```python
from build123d import *

# Parameters (mm, degrees)
SKETCH1_R               = 1.6
BOSS_EXTRUDE1_DEPTH     = 6
SALIENTE_EXTRUIR1_DEPTH = 7


with BuildPart() as part:
    # Sketch1 → Boss-Extrude1 (new body)
    # profile 1 of 2: a face of its own
    with BuildSketch(Plane.XY):
        with BuildLine():
            Line((31.98, 5), (0, 5))
            ThreePointArc((0, 5), (-5, 0), (0, -5))
            Line((0, -5), (33.93, -5))
            Line((33.93, -5), (37.237412205, -3.749803263))
            ThreePointArc((37.237412205, -3.749803263), (38.607019153, 1.767906062), (33.93, 5))
            Line((33.93, 5), (31.98, 5))
        make_face()
        Circle(SKETCH1_R, mode=Mode.SUBTRACT)
        with Locations((33.93, 0)):
            Circle(SKETCH1_R, mode=Mode.SUBTRACT)
    # profile 2 of 2: a face of its own
    with BuildSketch(Plane.XY):
        with BuildLine():
            Line((83.410038042, 35.902284495), (31.98, 5))
            Line((31.98, 5), (33.93, 5))
            ThreePointArc((33.93, 5), (38.607019153, 1.767906062), (37.237412205, -3.749803263))
            Line((37.237412205, -3.749803263), (88.667450247, 27.152481232))
            Line((88.667450247, 27.152481232), (83.410038042, 35.902284495))
        make_face()
    extrude(amount=BOSS_EXTRUDE1_DEPTH)

    # Croquis3 → Saliente-Extruir1 (add)
    with BuildSketch(Plane.XY.offset(6)):
        Polygon((83.410038042, 35.902284495), (88.667450247, 27.152481232), (54.380758219, 6.550958236), (49.123346014, 15.300761498), align=None)
    extrude(amount=SALIENTE_EXTRUIR1_DEPTH)


solid = part.part
```
Check sheet for the modelled part. Datum: model origin and axes. Units: mm. A direction names the side the tool comes from. Give positions to 0.01 mm unless a question says otherwise; leave off trailing zeros. Write each loop counter-clockwise with the first axis right and the second up, starting at its lowest first coordinate (ties: lowest second). Pieces come first, ordered by that corner, then holes.
Item 1: Cross-section at A-A (z = 3). Enter the section's corners in (x, y), and give its area (3 significant figures).
Item 2: Gauge pin test, flat ends, axial feed: pin 1 (3 mm diameter, centred on y = 30, z = 11.5, fed in from -X); pin 2 (2 mm diameter, centred on y = 19.5, z = 9, fed in from +X); pin 3 (16 mm diameter, centred on x = 35.5, y = 0.5, fed in from +Z). Record the tip position at first contact, or that the pin passes through.
Item 3: Cross-section at C-C (z = 9). Enter the section's corners in (x, y), and give its area (3 significant figures).
Item 4: Access from +Z, -Z, +X, -X, +Y, -Y to the whole of each face (thin tool, end or side, straight path). Record for faces 4 (the face through (69, 21, 13)), 5 (the face through (51.79, 10.86, 9.45)).
Item 5: Cross-section at D-D (y = 20). Enter the section's corners in (x, z), and give its area (3 significant figures).
Item 6: Draft check along Y on faces 1 (the face through (16, 5, 3)), 2 (the face through (17, -5, 3)), 3 (the face through (32.33, 0.07, 2.96)). Enter one of: released by +Y, released by -Y, zero draft, split by the parting line, or undercut.
Item 7: Scan lines: L1, parallel to Y at x = 0, z = 3.45; L2, parallel to Z at x = 27.5, y = 2; L3, parallel to Y at x = 33.93, z = 2.95. Record each from-to range of solid material in increasing order.
Item 8: Cross-section at B-B (y = 0). Enter the section's corners in (x, z), and give its area (3 significant figures).
Report:
1. outline: (0, -5) - (33.93, -5) - (37.24, -3.75) - (88.67, 27.15) - (83.41, 35.9) - (31.98, 5) - (0, 5) arc R5 ccw to start; hole circle Ø3.2 at (0, 0); hole circle Ø3.2 at (33.93, 0)
1. area: 983 mm2
2. pin 1: stops at x = 71.09
2. pin 2: stops at x = 77.6
2. pin 3: stops at z = 6
3. outline: (49.12, 15.3) - (54.38, 6.55) - (88.67, 27.15) - (83.41, 35.9) - close
3. area: 408 mm2
4. face 4: +Z, +X, -X, +Y, -Y
4. face 5: +Z, -X, -Y
5. outline: (56.94, 0) - (76.76, 0) - (76.76, 13) - (56.94, 13) - close
5. area: 258 mm2
6. face 1: released by +Y
6. face 2: released by -Y
6. face 3: undercut
7. L1: y = -5 to -1.6, 1.6 to 5
7. L2: z = 0 to 6
7. L3: y = -5 to -1.6, 1.6 to 6.17
8. outline: (-5, 0) - (-1.6, 0) - (-1.6, 6) - (-5, 6) - close; (1.6, 0) - (32.33, 0) - (32.33, 6) - (1.6, 6) - close; (35.53, 0) - (43.48, 0) - (43.48, 6) - (35.53, 6) - close
8. area: 252 mm2
